```python
from build123d import *

# Parameters (mm, degrees)
F0_W      = 43.434
F0_H      = 13.716
F1_DEPTH  = 16.657
F3_DEPTH  = 43.435
F4_W      = 4.5
F4_H      = 5
F5_DEPTH  = 6
F6_R      = 2.25
F7_DEPTH  = 2
F8_W      = 6
F8_H      = 0.75
F9_DEPTH  = 6.35
F10_W     = 6
F10_H     = 0.75
F11_DEPTH = 6.35
F12_R     = 2
F13_R     = 2
F14_DEPTH = 0.751
F15_R     = 2
F16_DEPTH = 0.751


# Not quite as in the source:
# - a feature names something its author has since deleted; it is built from what else it names


with BuildPart() as f1:
    # F0 (on Top) → F1 (new body)
    with BuildSketch(Plane.XY):
        Rectangle(F0_W, F0_H)
    extrude(amount=F1_DEPTH)

    # F2 (on face) → F3 (cut, through all)
    with BuildSketch(Plane(origin=(-21.717, 0, 0), x_dir=(0, -1, 0), z_dir=(-1, 0, 0))):
        Polygon((-6.858, 10.657), (-0.858, 16.657), (-6.858, 16.657), align=None)
        Polygon((6.858, 16.657), (-0.5295271985, 16.657), (0.5445904681, 14.1634047031), (4.491972737, 8.7391110137), (6.858, 6.0806702822), align=None)
    extrude(amount=-F3_DEPTH, mode=Mode.SUBTRACT)

    # F4 (on face) → F5 (cut)
    with BuildSketch(Plane.XZ.offset(6.858)):
        with Locations((-18.737, 6)):
            Rectangle(F4_W, F4_H)
        with Locations((-11.237, 6)):
            Rectangle(F4_W, F4_H)
        with Locations((-3.737, 6)):
            Rectangle(F4_W, F4_H)
        with Locations((3.763, 6)):
            Rectangle(F4_W, F4_H)
        with Locations((11.263, 6)):
            Rectangle(F4_W, F4_H)
        with Locations((18.763, 6)):
            Rectangle(F4_W, F4_H)
        with Locations((26.263, 6)):
            Rectangle(F4_W, F4_H)
        with Locations((33.763, 6)):
            Rectangle(F4_W, F4_H)
        with Locations((41.263, 6)):
            Rectangle(F4_W, F4_H)
        with Locations((48.763, 6)):
            Rectangle(F4_W, F4_H)
        with Locations((56.263, 6)):
            Rectangle(F4_W, F4_H)
        with Locations((63.763, 6)):
            Rectangle(F4_W, F4_H)
    extrude(amount=-F5_DEPTH, mode=Mode.SUBTRACT)

    # F6 (on face) → F7 (cut)
    with BuildSketch(Plane(origin=(0, 8.7575, 8.7575), x_dir=(1, 0, 0), z_dir=(0, 0.7071067812, 0.7071067812))):
        with Locations((-18.737, -6.9289393488)):
            Circle(F6_R)
        with Locations((-11.237, -6.9289393488)):
            Circle(F6_R)
        with Locations((-3.737, -6.9289393488)):
            Circle(F6_R)
        with Locations((3.763, -6.9289393488)):
            Circle(F6_R)
        with Locations((11.263, -6.9289393488)):
            Circle(F6_R)
        with Locations((18.763, -6.9289393488)):
            Circle(F6_R)
        with Locations((26.263, -6.9289393488)):
            Circle(F6_R)
        with Locations((33.763, -6.9289393488)):
            Circle(F6_R)
        with Locations((41.263, -6.9289393488)):
            Circle(F6_R)
        with Locations((48.763, -6.9289393488)):
            Circle(F6_R)
        with Locations((56.263, -6.9289393488)):
            Circle(F6_R)
        with Locations((63.763, -6.9289393488)):
            Circle(F6_R)
    extrude(amount=-F7_DEPTH, mode=Mode.SUBTRACT)

    # F8 (on face) → F9 (join)
    with BuildSketch(Plane(origin=(-21.717, 0, 0), x_dir=(0, -1, 0), z_dir=(-1, 0, 0))):
        with Locations((0, 0.375)):
            Rectangle(F8_W, F8_H)
    extrude(amount=F9_DEPTH)

    # F10 (on face) → F11 (join)
    with BuildSketch(Plane.YZ.offset(21.717)):
        with Locations((0, 0.375)):
            Rectangle(F10_W, F10_H)
    extrude(amount=F11_DEPTH)

    # F12
    f12_edges = [f1.edges().sort_by_distance(p)[0] for p in [
        (-28.067, 3, 0.375),
        (-28.067, -3, 0.375),
        (28.067, -3, 0.375),
        (28.067, 3, 0.375),
    ]]
    fillet(f12_edges, radius=F12_R)

    # F13 (on face) → F14 (cut, through all)
    with BuildSketch(Plane.XY.offset(0.75)):
        with Locations((-25.1435, 0)):
            Circle(F13_R)
    extrude(amount=-F14_DEPTH, mode=Mode.SUBTRACT)

    # F15 (on face) → F16 (cut, through all)
    with BuildSketch(Plane.XY.offset(0.75)):
        with Locations((25.1435, 0)):
            Circle(F15_R)
    extrude(amount=-F16_DEPTH, mode=Mode.SUBTRACT)


solid = f1.part
```
Can you work these out from the model? Positions are in its coordinate system, mm. A direction names the side the tool comes from. Round coordinates to 2 decimals unless told otherwise and drop trailing zeros. Loops run counter-clockwise (first coordinate to the right, second up) from the corner with the lowest first, then second, coordinate; pieces in that order, holes last. Notation, with made-up numbers: (-29, -11.75) -> (14, -11.75) arc R14 cw to (14, 11.25) -> close; hole circle Ø8 at (42.25, 56). An arc over 180 degrees is marked (long way). Answer in a Markdown table with one row per item.
Item 1: Suppose I cut it at A-A, the plane y = 0. List the corners of the cut face in (x, z) for me.
Answer block:
| item | result |
|---|---|
| outline | (-28.07, 0) -> (-27.14, 0) -> (-27.14, 0.75) -> (-28.07, 0.75) -> close; (-23.14, 0) -> (23.14, 0) -> (23.14, 0.75) -> (21.72, 0.75) -> (21.72, 15.43) -> (-21.72, 15.43) -> (-21.72, 0.75) -> (-23.14, 0.75) -> close; (27.14, 0) -> (28.07, 0) -> (28.07, 0.75) -> (27.14, 0.75) -> close |
Item 2: Suppose I cut it at C-C, the plane x = 17. List the corners of the cut face in (y, z) for me.
Answer block:
| item | result |
|---|---|
| outline | (-6.86, 0) -> (6.86, 0) -> (6.86, 10.66) -> (4.85, 12.67) -> (3.43, 11.25) -> (1.46, 13.23) -> (2.87, 14.65) -> (0.86, 16.66) -> (0.53, 16.66) -> (-0.54, 14.16) -> (-4.49, 8.74) -> (-4.7, 8.5) -> (-0.86, 8.5) -> (-0.86, 3.5) -> (-6.86, 3.5) -> close |
Item 3: On a 3-axis mill with a long thin cutter (end or side, diameter ignored), from which of +Z, -Z, +X, -X, +Y, -Y can I reach the whole of each face in a straight line? I mean faces 1 (the flat face through (-11.268, 2.466, 12.221)), 2 (the cylindrical face through (-23.296, -0.766, 0.38)), 3 (the flat face through (-5.987, -4, 6)). Say none if no direction works.
Answer block:
| item | result |
|---|---|
| face 1 | none |
| face 2 | +Z, -Z |
| face 3 | -Y |
Item 4: Will these pins go through, and if not, where does the flat tip stop? P1, Ø1.3, axis at x = -3.5, y = -3, coming from the +Z side; P2, Ø1.5, axis at y = -4, z = 7, coming from the +X side; P3, Ø2.5, axis at y = -3.5, z = 6, coming from the -X side.
Answer block:
| item | result |
|---|---|
| P1 | z = 11.68 |
| P2 | x = 21.72 |
| P3 | x = -21.72 |
Item 5: We'd pull the mould along Z, two halves only. Please class faces 4 (the flat face through (-23, 1, 0.75)), 5 (the cylindrical face through (13.34, 2.55, 13.57)), 6 (the cylindrical face through (27.466, -2.43, 0.38)): released by +Z, released by -Z, zero draft, split by the parting line, or undercut.
Answer block:
| item | result |
|---|---|
| face 4 | released by +Z |
| face 5 | undercut |
| face 6 | zero draft |
Item 6: If I drill on probe 1 along X at (y, z) = (5, 1); probe 2 along Y at (x, z) = (-4, 11.75) (3 decimals); probe 3 along Z at (x, y) = (-19, 1.5) (3 decimals), over which ranges is the centre line in solid material (lowest first)?
Answer block:
| item | result |
|---|---|
| probe 1 | -21.72 to 21.72 |
| probe 2 | -2.301 to 2.937, 5.111 to 5.765 |
| probe 3 | 0 to 13.187, 14.459 to 16.015 |
Item 7: Suppose I cut it at B-B, the plane x = -15. List the corners of the cut face in (y, z) for me.
Answer block:
| item | result |
|---|---|
| outline | (-6.86, 0) -> (6.86, 0) -> (6.86, 10.66) -> (0.86, 16.66) -> (0.53, 16.66) -> (-0.54, 14.16) -> (-4.49, 8.74) -> (-6.86, 6.08) -> close |
